from build123d import *

# Parameters (mm, degrees)
F0_W      = 140
F0_H      = 80
F0_W_2    = 130
F0_H_2    = 70
F1_DEPTH  = 70
F2_DEPTH  = 5
F3_W      = 5
F3_H      = 70
F4_DEPTH  = 5
F6_DEPTH  = 2
F8_DEPTH  = 2
F10_DEPTH = 2
F11_R     = 2.99999
F12_R     = 1.5
F13_DEPTH = 1


# Not quite as in the source:
# - a fillet or chamfer is up to 0.001 mm smaller than in the source, because OpenCascade refuses the exact size


with BuildPart() as f1:
    # F0 (on Top) → F1 (new body)
    with BuildSketch(Plane.XY):
        Rectangle(F0_W, F0_H)
        Rectangle(F0_W_2, F0_H_2, mode=Mode.SUBTRACT)
    extrude(amount=F1_DEPTH)

    # F0 (on Top) → F2 (join)
    with BuildSketch(Plane.XY):
        Rectangle(F0_W_2, F0_H_2)
    extrude(amount=F2_DEPTH)

    # F3 (on face) → F4 (cut)
    with BuildSketch(Plane.XY.offset(70)):
        with Locations((67.5, 0)):
            Rectangle(F3_W, F3_H)
    extrude(amount=-F4_DEPTH, mode=Mode.SUBTRACT)

    # F5 (on face) → F6 (cut)
    with BuildSketch(Plane.XZ.offset(-35)):
        Polygon((65, 65), (70, 65), (70, 68), (-65, 68), (-65, 65), align=None)
    extrude(amount=-F6_DEPTH, mode=Mode.SUBTRACT)

    # F7 (on face) → F8 (cut)
    with BuildSketch(Plane.YZ.offset(-65)):
        Polygon((35, 65), (37, 65), (37, 68), (35, 68), (-35, 68), (-35, 65), align=None)
    extrude(amount=-F8_DEPTH, mode=Mode.SUBTRACT)

    # F9 (on face) → F10 (cut)
    with BuildSketch(Plane(origin=(0, -35, 0), x_dir=(-1, 0, 0), z_dir=(0, 1, 0))):
        Polygon((65, 65), (67, 65), (67, 68), (65, 68), (-70, 68), (-70, 65), (-65, 65), align=None)
    extrude(amount=-F10_DEPTH, mode=Mode.SUBTRACT)

    # F11 (radius 3 in the source; OpenCascade refuses exactly that, so slightly less here)
    f11_edges = [f1.edges().sort_by_distance(p)[0] for p in [
        (-70, -40, 35),
        (-70, 40, 35),
        (70, 40, 35),
        (70, -40, 35),
    ]]
    fillet(f11_edges, radius=F11_R)

    # F12
    f12_edges = [f1.edges().sort_by_distance(p)[0] for p in [
        (-67, -37, 66.5),
        (-67, 37, 66.5),
    ]]
    fillet(f12_edges, radius=F12_R)

    # F13 (add): a face of the model
    f13_faces = [f1.faces().sort_by_distance(p)[0] for p in [
        (-68.3875484503, 0, 70),
    ]]
    extrude(f13_faces, amount=F13_DEPTH)


solid = f1.part
The model under review builds one solid part; all positions refer to its coordinate system, in mm. A direction names the side the tool comes from. Round coordinates to 2 decimals unless told otherwise and drop trailing zeros. Order: outer loops, then holes, each group sorted by start corner. A loop starts at its lowest first (then second) coordinate and runs counter-clockwise, first axis right, second up. Notation, with made-up numbers: (-5.5, 83) -> (1.5, 83) arc R14 cw to (1.5, 103) -> close; hole circle Ø10 at (75, 50). An arc over 180 degrees is marked (long way). Return JSON: item names as keys, results as strings.
1. Take a section at B-B (x = 42.5). Write out the cut boundary in (y, z), then the cut area to 3 significant figures.
Answer block:
{"outline": "(-40, 0) -> (40, 0) -> (40, 71) -> (35, 71) -> (35, 68) -> (37, 68) -> (37, 65) -> (35, 65) -> (35, 5) -> (-35, 5) -> (-35, 65) -> (-37, 65) -> (-37, 68) -> (-35, 68) -> (-35, 71) -> (-40, 71) -> close", "area": "1,050 mm²"}
2. The part is to be moulded in two halves that separate along Y. For faces 5 (the face through (-1, 40, 35)), 6 (the face through (2, -36, 68)), 7 (the face through (69.14, -39.1, 36)), say which applies: +Y half, -Y half, draft (parallel to the pull), parting line (faces both ways), or undercut.
Answer block:
{"face 5": "+Y half", "face 6": "undercut", "face 7": "-Y half"}
3. For faces 1 (the face through (-65, 0, 69)), 2 (the face through (-70, -1, 35)), 3 (the face through (21.5, 35.5, 65)), 4 (the face through (-1, 35, 35)), list the 3-axis set-ups (+Z, -Z, +X, -X, +Y, -Y) from which the entire face can be reached by the end or side of a thin tool; tool diameter is ignored.
Answer block:
{"face 1": "+Z, +X", "face 2": "+Z, -Z, -X, +Y, -Y", "face 3": "+X", "face 4": "+Z"}
4. Take a section at C-C (y = 32). Write out the cut boundary in (x, z), then the cut area to 3 significant figures.
Answer block:
{"outline": "(-70, 0) -> (70, 0) -> (70, 65) -> (65, 65) -> (65, 5) -> (-65, 5) -> (-65, 65) -> (-67, 65) -> (-67, 68) -> (-65, 68) -> (-65, 71) -> (-70, 71) -> close", "area": "1,320 mm²"}
5. For L1, parallel to X at y = 32, z = 19; L2, parallel to Y at x = -14, z = 23; L3, parallel to Z at x = 35.5, y = 25.5, list the stretches that pass through material, from the lowest coordinate up. Write a range as [from, to].
Answer block:
{"L1": "x = [-70, -65], [65, 70]", "L2": "y = [-40, -35], [35, 40]", "L3": "z = [0, 5]"}
6. Take a section at A-A (z = 60). Write out the cut boundary in (x, y).
Answer block:
{"outline": "(-70, -37) arc R3 ccw to (-67, -40) -> (67, -40) arc R3 ccw to (70, -37) -> (70, 37) arc R3 ccw to (67, 40) -> (-67, 40) arc R3 ccw to (-70, 37) -> close; hole (-65, -35) -> (65, -35) -> (65, 35) -> (-65, 35) -> close"}
7. Insertion check: P1, Ø5, axis at x = 1.5, y = 25.5, coming from the -Z side; P2, Ø8, axis at x = 15, y = 25, coming from the +Z side; P3, Ø2.5, axis at y = -1, z = 69, coming from the +X side; P4, Ø1.5, axis at y = 1, z = 67, coming from the +X side. Each pin has a flat end and moves straight along its axis. Give the tip position at first contact, or say it passes through.
Answer block:
{"P1": "stops at z = 0", "P2": "stops at z = 5", "P3": "stops at x = -65", "P4": "stops at x = -67"}
